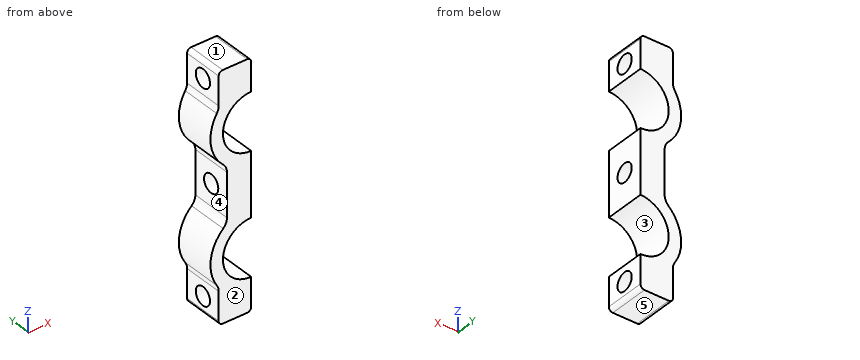
from build123d import *

# Parameters (mm, degrees)
EXTRUDE_1_DEPTH          = 10
EXTRUDE_2_DEPTH          = 10
SKETCH_3_R               = 2.25
CUT_EXTRUDE_1_DEPTH      = 5.049845
CUT_EXTRUDE_1_DEPTH_BACK = 4
EXTRUDE_4_DEPTH          = 10
SKETCH_4_R               = 2.25
CUT_EXTRUDE_2_DEPTH      = 7
FILLET_1_R               = 3
FILLET_2_R               = 1
EXTRUDE_3_DEPTH          = 10
FILLET_3_R               = 1


with BuildPart() as part:
    # Эскиз1 → Бобышка-Вытянуть1 (new body)
    with BuildSketch(Plane(origin=(0, 0, 0), x_dir=(1, 0, 0), z_dir=(0, 1, 0))):
        with BuildLine():
            Line((0, 0), (0, 8))
            ThreePointArc((0, 8), (-7.1, 15.1), (0, 22.2))
            Line((0, 22.2), (0, 37.8))
            ThreePointArc((0, 37.8), (-7.1, 44.9), (0, 52))
            Line((0, 52), (0, 60))
            Line((0, 60), (-3, 60))
            Line((-3, 60), (-3, 54.544169223))
            ThreePointArc((-3, 54.544169223), (-10.1, 44.9), (-3, 35.255830777))
            Line((-3, 35.255830777), (-3, 24.744169223))
            ThreePointArc((-3, 24.744169223), (-10.1, 15.1), (-3, 5.455830777))
            Line((-3, 5.455830777), (-3, 0))
            Line((-3, 0), (0, 0))
        make_face()
    extrude(amount=EXTRUDE_1_DEPTH)

    # Эскиз2 → Бобышка-Вытянуть2 (add)
    with BuildSketch(Plane(origin=(0, 10, 0), x_dir=(1, 0, 0), z_dir=(0, 1, 0))):
        with BuildLine():
            Line((-3, 60), (-8.049844719, 60))
            Line((-8.049844719, 60), (-8.049844719, 51))
            ThreePointArc((-8.049844719, 51), (-5.802159163, 53.167100402), (-3, 54.544169223))
            Line((-3, 54.544169223), (-3, 60))
        make_face()
        with BuildLine():
            Line((-3, 0), (-3, 5.455830777))
            ThreePointArc((-3, 5.455830777), (-5.802159163, 6.832899598), (-8.049844719, 9))
            Line((-8.049844719, 9), (-8.049844719, 0))
            Line((-8.049844719, 0), (-3, 0))
        make_face()
    extrude(amount=-EXTRUDE_2_DEPTH)

    # Эскиз3 → Вырез-Вытянуть1 (cut, two sides)
    with BuildSketch(Plane.ZY.offset(3)) as cut_extrude_1_sk:
        with Locations((-55.75, 5)):
            Circle(SKETCH_3_R)
        with Locations((-4.25, 5)):
            Circle(SKETCH_3_R)
    extrude(amount=CUT_EXTRUDE_1_DEPTH, mode=Mode.SUBTRACT)
    extrude(cut_extrude_1_sk.sketch, amount=-CUT_EXTRUDE_1_DEPTH_BACK, mode=Mode.SUBTRACT)

    # Эскиз7 → Бобышка-Вытянуть4 (add, through all)
    with BuildSketch(Plane(origin=(-3, 0, 0), x_dir=(0, 0, 1), z_dir=(0, 1, 0))):
        with BuildLine():
            Line((-36.775346161, -3), (-23.224653839, -3))
            ThreePointArc((-23.224653839, -3), (-24.11014807, -1.563686202), (-24.744169223, 0))
            Line((-24.744169223, 0), (-35.255830777, 0))
            ThreePointArc((-35.255830777, 0), (-35.88985193, -1.563686202), (-36.775346161, -3))
        make_face()
    extrude(amount=EXTRUDE_4_DEPTH)

    # Эскиз4 → Вырез-Вытянуть2 (cut, through all)
    with BuildSketch(Plane.ZY.offset(6)):
        with Locations((-30, 5)):
            Circle(SKETCH_4_R)
    extrude(amount=-CUT_EXTRUDE_2_DEPTH, mode=Mode.SUBTRACT)

    # Скругление1
    fillet_1_edges = [part.edges().sort_by_distance(p)[0] for p in [
        (-8.049844719, 5, -51),
        (-8.049844719, 5, -9),
        (-6, 5, -36.775346161),
        (-6, 5, -23.224653839),
    ]]
    fillet(fillet_1_edges, radius=FILLET_1_R)

    # Скругление2
    fillet_2_edges = [part.edges().sort_by_distance(p)[0] for p in [
        (-8.049844719, 5, -60),
        (-8.049844719, 5, 0),
    ]]
    fillet(fillet_2_edges, radius=FILLET_2_R)

    # Эскиз5 → Бобышка-Вытянуть3 (add, through all)
    with BuildSketch(Plane.XZ):
        with BuildLine():
            Line((0, -8), (0, -8.1))
            ThreePointArc((0, -8.1), (-7, -15.1), (0, -22.1))
            Line((0, -22.1), (0, -22.2))
            ThreePointArc((0, -22.2), (-7.1, -15.1), (0, -8))
        make_face()
        with BuildLine():
            Line((0, -51.9), (0, -52))
            ThreePointArc((0, -52), (-7.1, -44.9), (0, -37.8))
            Line((0, -37.8), (0, -37.9))
            ThreePointArc((0, -37.9), (-7, -44.9), (0, -51.9))
        make_face()
    extrude(amount=-EXTRUDE_3_DEPTH)

    # Скругление3
    fillet_3_edges = [part.edges().sort_by_distance(p)[0] for p in [
        (0, 5, -60),
        (0, 5, 0),
    ]]
    fillet(fillet_3_edges, radius=FILLET_3_R)


solid = part.part
Verification items for the finished model (mm, model axes). Face numbers are marked on the shaded views. A direction names the side the tool comes from. Coordinates: 2 decimals unless noted, no trailing zeros. Order: outer loops, then holes, each group sorted by start corner. A loop starts at its lowest first (then second) coordinate and runs counter-clockwise, first axis right, second up. Notation, with made-up numbers: M 31.5,-1 L 41.5,-1 A19 ccw 41.5,29 Z; hole C 59,65 d3. An arc over 180 degrees is marked long. One line per item, written item: value. Start each with the question number.
Item 1: Sectioned sample at A-A (y = 5). Count the separate pieces of the cut face and the enclosed holes in it, then the cut area to 3 significant figures.
Item 2: Sectioned sample at C-C (x = -4.5). Enter the section's corners in (y, z), then the cut area to 3 significant figures.
Item 3: Mould release check, pull along Z, two halves, no side actions. Record for the marked faces 1, 2 and 3: released by +Z, released by -Z, zero draft, split by the parting line, or undercut.
Item 4: Sectioned sample at D-D (y = 1.25). Enter the section's corners in (x, z).
Item 5: Gauge pin test, flat ends, axial feed: pin 1 (1.5 mm diameter, centred on x = -8.5, y = 9, fed in from -Z); pin 2 (6 mm diameter, centred on y = 5, z = -55.75, fed in from +X); pin 3 (5 mm diameter, centred on y = 6, z = -12, fed in from -X); pin 4 (2.5 mm diameter, centred on y = 5, z = -55.75, fed in from -X). Record the tip position at first contact, or that the pin passes through.
Item 6: Sectioned sample at B-B (z = -4.25). Enter the section's corners in (x, y).
Item 7: Access from +Z, -Z, +X, -X, +Y, -Y to the whole of each face (thin tool, end or side, straight path). Record for the marked faces 4 and 5.
Item 8: Scan lines: probe 1 along Y at (x, z) = (-0.75, -30); probe 2 along Z at (x, y) = (-2.75, 6); probe 3 along X at (y, z) = (2.75, -26). Record each from-to range of solid material in increasing order.
Conclusion:
1. separate pieces: 4
1. enclosed holes: 0
1. area: 232 mm^2
2. outline: M 0,-60 L 10,-60 L 10,-50.26 L 0,-50.26 Z; M 0,-39.54 L 10,-39.54 L 10,-20.46 L 0,-20.46 Z; M 0,-9.74 L 10,-9.74 L 10,0 L 0,0 Z; hole C 5,-55.75 d4.5; hole C 5,-30 d4.5; hole C 5,-4.25 d4.5
2. area: 338 mm^2
3. face 1: released by +Z
3. face 2: zero draft
3. face 3: undercut
4. outline: M -8.52,-50.33 A3 cw -8.05,-51.94 L -8.05,-59 A1 ccw -7.05,-60 L -1,-60 A1 ccw 0,-59 L 0,-51.9 A7 cw 0,-37.9 L 0,-22.1 A7 cw 0,-8.1 L 0,-1 A1 ccw -1,0 L -7.05,0 A1 ccw -8.05,-1 L -8.05,-8.06 A3 cw -8.52,-9.67 A10.1 ccw -6.94,-22.44 A3 cw -6,-24.62 L -6,-35.38 A3 cw -6.94,-37.56 A10.1 ccw Z
5. pin 1: stops at z = -59.71
5. pin 2: stops at x = 0
5. pin 3: stops at x = -10.08
5. pin 4: passes through
6. outline: M -8.05,0 L 0,0 L 0,2.75 L -8.05,2.75 Z; M -8.05,7.25 L 0,7.25 L 0,10 L -8.05,10 Z
7. face 4: -X, +Y, -Y
7. face 5: -Z, +X, -X, +Y, -Y
8. probe 1: y = 0 to 2.75, 7.25 to 10
8. probe 2: z = -60 to -57.77, -53.73 to -51.34, -38.46 to -32.02, -27.98 to -21.54, -8.66 to -6.27, -2.23 to 0
8. probe 3: x = -6 to 0
